For this review, take the finished solid that the model builds, in its own axes (mm). Face numbers are marked on the shaded views. A direction names the side the tool comes from. Give positions to 0.01 mm unless a question says otherwise; leave off trailing zeros. Write each loop counter-clockwise with the first axis right and the second up, starting at its lowest first coordinate (ties: lowest second). Pieces come first, ordered by that corner, then holes. Notation, with made-up numbers: (52, -21.5) -> (106, -21.5) arc R14 cw to (106, -3.5) -> close; hole circle Ø11 at (-4, -30). An arc over 180 degrees is marked (long way). Write item = value, one per line.
```python
from build123d import *

# Parameters (mm, degrees)
F0_W     = 46.99
F0_H     = 33.02
F1_DEPTH = 71.12
F3_DEPTH = 86.36
F5_W     = 86.868
F5_H     = 58.928
F6_DEPTH = 65.532


with BuildPart() as f1:
    # F0 (on Top) → F1 (new body)
    with BuildSketch(Plane.XY):
        with Locations((-23.495, -16.51)):
            Rectangle(F0_W, F0_H)
        Polygon((0, 0), (0, -33.02), (46.99, -33.02), (46.99, 33.02), (-46.99, 33.02), (-46.99, 0), align=None)
    extrude(amount=F1_DEPTH)

    # F2 (on face) → F3 (join)
    with BuildSketch(Plane(origin=(0, 33.02, 0), x_dir=(-1, 0, 0), z_dir=(0, 1, 0))):
        with BuildLine():
            ThreePointArc((49.0112789095, 31.9781005383), (48.6423795188, 33.0874779076), (49.1006532674, 34.1630196685))
            Line((49.1006532674, 34.1630196685), (46.99, 34.1630196685))
            Line((46.99, 34.1630196685), (46.99, 31.9781005383))
            Line((46.99, 31.9781005383), (49.0112789095, 31.9781005383))
        make_face()
        with BuildLine():
            Line((49.1006532674, 31.9781005383), (49.1006532674, 34.1630196685))
            ThreePointArc((49.1006532674, 34.1630196685), (48.6423795188, 33.0874779076), (49.0112789095, 31.9781005383))
            Line((49.0112789095, 31.9781005383), (49.1006532674, 31.9781005383))
        make_face()
        with BuildLine():
            ThreePointArc((49.0112789095, 31.9781005383), (50.8448700026, 31.464321447), (51.943, 33.02))
            ThreePointArc((51.943, 33.02), (50.9079900748, 34.5517823696), (49.1006532674, 34.1630196685))
            Line((49.1006532674, 34.1630196685), (49.1006532674, 31.9781005383))
            Line((49.1006532674, 31.9781005383), (49.0112789095, 31.9781005383))
        make_face()
    extrude(amount=-F3_DEPTH)

    # F4: F1 across plane


with BuildPart() as f1_1:
    add(f1.part)
    add(f1.part.mirror(Plane.YZ))

    # F5 (on face) → F6 (cut)
    with BuildSketch(Plane.XY.offset(71.12)):
        Rectangle(F5_W, F5_H)
    extrude(amount=-F6_DEPTH, mode=Mode.SUBTRACT)


solid = f1_1.part
```
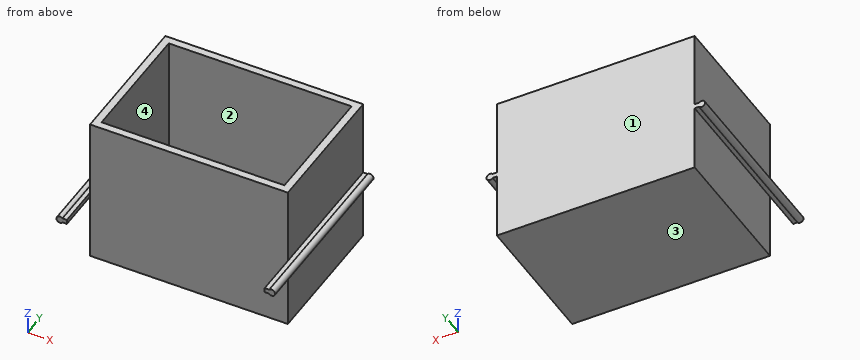
(1) For pin 1 (1.5 mm diameter, centred on y = 7.5, z = 41, fed in from +X); pin 2 (0.6 mm diameter, centred on x = -48, y = 8.5, fed in from +Z); pin 3 (0.6 mm diameter, centred on x = -47.5, y = -29, fed in from -Z), all flat-tipped, find the tip position at first contact; note any pin that passes through.
Answers below:
pin_1 = 46.99
pin_2 = 34.16
pin_3 = 31.98
(2) Take a section at A-A (z = 67). Write out the cut boundary in (x, y), plus the area to 3 significant figures.
Answers below:
outline = (-46.99, -33.02) -> (46.99, -33.02) -> (46.99, 33.02) -> (-46.99, 33.02) -> close; hole (-43.43, -29.46) -> (43.43, -29.46) -> (43.43, 29.46) -> (-43.43, 29.46) -> close
area = 1,090 mm^2
(3) The part is to be moulded in two halves that separate along X. For the marked faces 1 and 2, say which applies: released by +X, released by -X, zero draft, split by the parting line, or undercut.
Answers below:
face_1 = zero draft
face_2 = undercut
(4) Take a section at C-C (y = 21). Write out the cut boundary in (x, z), plus the area to 3 significant figures.
Answers below:
outline = (-49.1, 34.16) arc R1.65 ccw (long way) to (-49.01, 31.98) -> (-46.99, 31.98) -> (-46.99, 0) -> (46.99, 0) -> (46.99, 31.98) -> (49.01, 31.98) arc R1.65 ccw (long way) to (49.1, 34.16) -> (46.99, 34.16) -> (46.99, 71.12) -> (43.43, 71.12) -> (43.43, 5.59) -> (-43.43, 5.59) -> (-43.43, 71.12) -> (-46.99, 71.12) -> (-46.99, 34.16) -> close
area = 1,020 mm^2
(5) To check wall thickness, follow probe 1 along X at (y, z) = (26, 67.5); probe 2 along Y at (x, z) = (21.5, 18.5); probe 3 along Z at (x, y) = (21, -27). State the ranges of each line that lie inside material, in increasing order.
Answers below:
probe_1 = -46.99 to -43.43, 43.43 to 46.99
probe_2 = -33.02 to -29.46, 29.46 to 33.02
probe_3 = 0 to 5.59
(6) Take a section at B-B (y = -47). Write out the cut boundary in (x, z).
Answers below:
outline = (-49.1, 34.16) arc R1.65 ccw (long way) to (-49.01, 31.98) -> (-46.99, 31.98) -> (-46.99, 34.16) -> close; (46.99, 31.98) -> (49.01, 31.98) arc R1.65 ccw (long way) to (49.1, 34.16) -> (46.99, 34.16) -> close
(7) Tool access review of the marked faces 3 and 4: name each direction out of +Z, -Z, +X, -X, +Y, -Y from which nothing blocks a thin tool from reaching the whole face with its end or side.
Answers below:
face_3 = -Z, +X, -X, +Y, -Y
face_4 = +Z
(8) Take a section at D-D (x = -20.5). Write out the cut boundary in (y, z), plus the area to 3 significant figures.
Answers below:
outline = (-33.02, 0) -> (33.02, 0) -> (33.02, 71.12) -> (29.46, 71.12) -> (29.46, 5.59) -> (-29.46, 5.59) -> (-29.46, 71.12) -> (-33.02, 71.12) -> close
area = 835 mm^2
